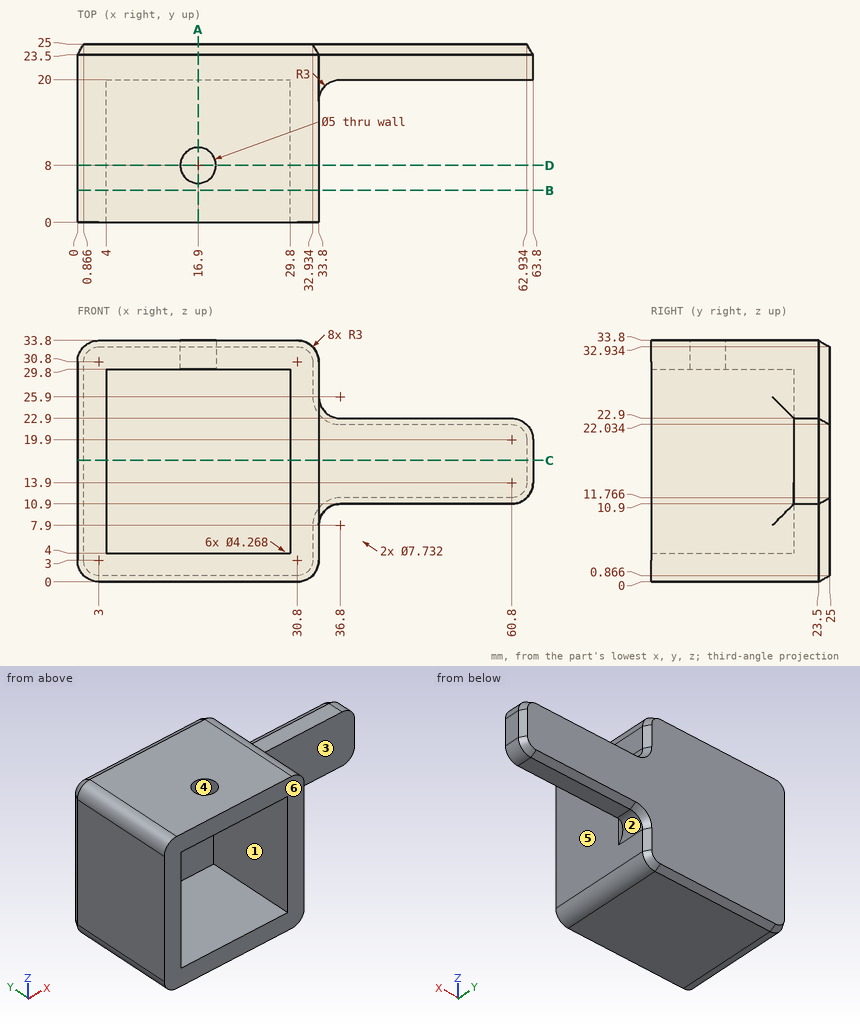
Design review of the part shown in the three views and the two pictorial views. Dimensions are in mm from the part's minimum x, y and z. A direction names the side the tool comes from. Give positions to 0.01 mm unless a question says otherwise; leave off trailing zeros. Write each loop counter-clockwise with the first axis right and the second up, starting at its lowest first coordinate (ties: lowest second). Pieces come first, ordered by that corner, then holes.
Item 1: Wall thickness on probe 1 along Y at (x, z) = (16.9, 32.8); probe 2 along X at (y, z) = (4.75, 14): over which ranges is each line inside the solid? List them lowest first.
Item 2: Insertion check: P1, Ø1, axis at x = 40.5, y = 20.5, coming from the -Z side; P2, Ø10, axis at y = 13, z = 13.5, coming from the -X side; P3, Ø1.5, axis at y = 17, z = 11, coming from the +X side; P4, Ø3, axis at x = 39, y = 19, coming from the +Z side. Each pin has a flat end and moves straight along its axis. Give the tip position at first contact, or say it passes through.
Item 3: Take a section at A-A (x = 16.9). Give the boundary of the cut face in (y, z), and give its area (3 significant figures).
Item 4: Take a section at D-D (y = 8). Give the boundary of the cut face in (x, z), and give its area (3 significant figures).
Item 5: Machinability: for the marked faces 1, 2 and 3, which of the approach directions +Z, -Z, +X, -X, +Y, -Y give a long, thin tool a straight path to every point of the face, cutting with its end or side? Answer none if there is none.
Item 6: Take a section at C-C (z = 17). Give the boundary of the cut face in (x, y), and give its area (3 significant figures).
Item 7: The part is to be moulded in two halves that separate along X. For the marked faces 4, 5 and 6, say which applies: +X half, -X half, draft (parallel to the pull), parting line (faces both ways), or undercut.
Item 8: Take a section at B-B (y = 4.5). Give the boundary of the cut face in (x, z).
Established:
1. probe 1: y = 0 to 5.5, 10.5 to 25
1. probe 2: x = 0 to 4, 29.8 to 33.8
2. P1: stops at z = 10.9
2. P2: stops at x = 0
2. P3: stops at x = 33.9
2. P4: stops at z = 22.9
3. outline: (0, 0) - (23.5, 0) - (25, 0.87) - (25, 32.93) - (23.5, 33.8) - (10.5, 33.8) - (10.5, 29.8) - (20, 29.8) - (20, 4) - (0, 4) - close; (0, 29.8) - (5.5, 29.8) - (5.5, 33.8) - (0, 33.8) - close
3. area: 308 mm2
4. outline: (0, 3) arc R3 ccw to (3, 0) - (30.8, 0) arc R3 ccw to (33.8, 3) - (33.8, 30.8) arc R3 ccw to (30.8, 33.8) - (19.4, 33.8) - (19.4, 29.8) - (29.8, 29.8) - (29.8, 4) - (4, 4) - (4, 29.8) - (14.4, 29.8) - (14.4, 33.8) - (3, 33.8) arc R3 ccw to (0, 30.8) - close
4. area: 449 mm2
5. face 1: -Y
5. face 2: -Z, +X, +Y, -Y
5. face 3: +Z, -Z, +X, -Y
6. outline: (0, 0) - (4, 0) - (4, 20) - (29.8, 20) - (29.8, 0) - (33.8, 0) - (33.8, 17) arc R3 cw to (36.8, 20) - (63.8, 20) - (63.8, 23.5) - (62.93, 25) - (0.87, 25) - (0, 23.5) - close
6. area: 480 mm2
7. face 4: undercut
7. face 5: +X half
7. face 6: draft
8. outline: (0, 3) arc R3 ccw to (3, 0) - (30.8, 0) arc R3 ccw to (33.8, 3) - (33.8, 30.8) arc R3 ccw to (30.8, 33.8) - (3, 33.8) arc R3 ccw to (0, 30.8) - close; hole (4, 4) - (29.8, 4) - (29.8, 29.8) - (4, 29.8) - close
